Read the model definition and answer for the solid it produces. Units are mm, in the model's axes. Coordinates: 2 decimals unless noted, no trailing zeros. Write each loop counter-clockwise with the first axis right and the second up, starting at its lowest first coordinate (ties: lowest second). Pieces come first, ordered by that corner, then holes.
Item 1: Section C-C (y = 9) is taken. Give the vertices of the cut face in (x, z).
Item 2: Section B-B (z = 2.5) is taken. Give the vertices of the cut face in (x, y) (3 decimals), then the cut area to 3 significant figures.
Item 3: Section A-A (x = 0) is taken. State how many separate pieces and enclosed holes the cut face has, then the cut area to 3 significant figures.
Item 4: Each of these flat-tipped pins is pushed along its axis until it touches: P1, Ø1.6, axis at y = 5.5, z = -26.5, coming from the -X side; P2, Ø2.5, axis at x = 2.5, z = 34.5, coming from the +Y side (3 decimals); P3, Ø4, axis at x = -1.5, z = -0.5, coming from the +Y side. Where does it stop, or does it pass through?
Item 5: Straight lines are drawn through the part: probe 1 along Z at (x, y) = (0, 6.8); probe 2 along X at (y, z) = (1.5, 17) (3 decimals); probe 3 along Z at (x, y) = (-0.25, 3). For each, find the intervals that lie inside material, in ascending order.
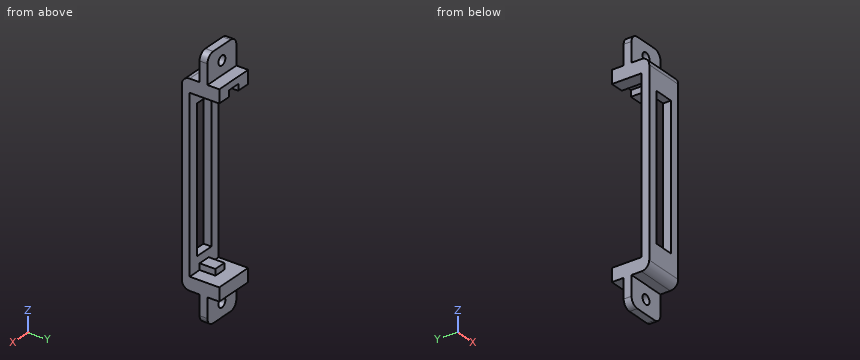
from build123d import *

# Parameters (mm, degrees)
SKETCH1_W           = 12.7
SKETCH1_H           = 63.5
SKETCH1_W_2         = 6.35
SKETCH1_H_2         = 45.72
BOSS_EXTRUDE1_DEPTH = 2.54
BOSS_EXTRUDE2_DEPTH = 9.525
SKETCH5_W           = 3.9878
SKETCH5_H           = 2.0066
CUT_EXTRUDE1_DEPTH  = 4.445
SKETCH7_W           = 12.7
SKETCH7_H           = 8.89
SKETCH7_R           = 1.524
BOSS_EXTRUDE4_DEPTH = 2.54
FILLET1_R           = 2.54


with BuildPart() as part:
    # Sketch1 → Boss-Extrude1 (new body)
    with BuildSketch(Plane(origin=(0, 0, 0), x_dir=(1, 0, 0), z_dir=(0, 1, 0))):
        Rectangle(SKETCH1_W, SKETCH1_H)
        Rectangle(SKETCH1_W_2, SKETCH1_H_2, mode=Mode.SUBTRACT)
    extrude(amount=BOSS_EXTRUDE1_DEPTH)

    # Sketch2 → Boss-Extrude2 (add)
    with BuildSketch(Plane(origin=(0, 2.54, 0), x_dir=(1, 0, 0), z_dir=(0, 1, 0))):
        Polygon((-6.35, 31.75), (6.35, 31.75), (6.35, 27.4955), (1.9939, 27.4955), (1.9939, 25.4889), (-1.9939, 25.4889), (-1.9939, 27.4955), (-6.35, 27.4955), align=None)
        Polygon((-6.35, -27.4955), (-6.35, -31.75), (6.35, -31.75), (6.35, -27.4955), (1.9939, -27.4955), (1.9939, -29.5021), (-1.9939, -29.5021), (-1.9939, -27.4955), align=None)
    extrude(amount=BOSS_EXTRUDE2_DEPTH)

    # Sketch5 → Cut-Extrude1 (cut)
    with BuildSketch(Plane(origin=(0, 12.065, 0), x_dir=(1, 0, 0), z_dir=(0, 1, 0))):
        with Locations((0, 26.4922)):
            Rectangle(SKETCH5_W, SKETCH5_H)
    extrude(amount=-CUT_EXTRUDE1_DEPTH, mode=Mode.SUBTRACT)

    # Sketch7 → Boss-Extrude4 (add)
    with BuildSketch(Plane(origin=(0, 8.255, 0), x_dir=(1, 0, 0), z_dir=(0, 1, 0))):
        with Locations((0, 36.195)):
            Rectangle(SKETCH7_W, SKETCH7_H)
        with Locations((0, 36.195)):
            Circle(SKETCH7_R, mode=Mode.SUBTRACT)
        with Locations((0, -36.195)):
            Rectangle(SKETCH7_W, SKETCH7_H)
        with Locations((0, -36.195)):
            Circle(SKETCH7_R, mode=Mode.SUBTRACT)
    extrude(amount=-BOSS_EXTRUDE4_DEPTH)

    # Fillet1
    fillet1_edges = [part.edges().sort_by_distance(p)[0] for p in [
        (6.35, 6.985, 40.64),
        (-6.35, 6.985, 40.64),
        (0, 0, 31.75),
        (0, 0, -31.75),
        (6.35, 6.985, -40.64),
        (-6.35, 6.985, -40.64),
    ]]
    fillet(fillet1_edges, radius=FILLET1_R)


solid = part.part
Established:
1. outline: (-6.35, -31.75) - (6.35, -31.75) - (6.35, -27.5) - (-6.35, -27.5) - close; (-6.35, 27.5) - (-1.99, 27.5) - (-1.99, 29.5) - (1.99, 29.5) - (1.99, 27.5) - (6.35, 27.5) - (6.35, 31.75) - (-6.35, 31.75) - close
2. outline: (-6.35, 0) - (-3.175, 0) - (-3.175, 2.54) - (-6.35, 2.54) - close; (3.175, 0) - (6.35, 0) - (6.35, 2.54) - (3.175, 2.54) - close
2. area: 16.1 mm2
3. separate pieces: 4
3. enclosed holes: 0
3. area: 144 mm2
4. P1: stops at x = -1.99
4. P2: stops at y = 8.255
4. P3: stops at y = 2.54
5. probe 1: z = -40.64 to -37.72, -34.67 to -25.49, 29.5 to 34.67, 37.72 to 40.64
5. probe 2: x = -6.35 to -3.175, 3.175 to 6.35
5. probe 3: z = -31.75 to -25.49, 29.5 to 31.75
